Could you check a few things on this model? Use its own coordinates, in mm. A direction names the side the tool comes from. Round coordinates to 2 decimals unless told otherwise and drop trailing zeros. Write each loop counter-clockwise with the first axis right and the second up, starting at its lowest first coordinate (ties: lowest second). Pieces come first, ordered by that corner, then holes.
```python
from build123d import *

# Parameters (mm, degrees)
EXTRUDE_1_DEPTH        = 65
EXTRUDE_2_DEPTH        = 5
EXTRUDE_3_DEPTH        = 8
SKETCH_8_R             = 2.3
CUT_EXTRUDE_4_DEPTH    = 3.5
CUT_EXTRUDE_6_DEPTH    = 14
EXTRUDE_4_DEPTH        = 40
HOLE_WIZARD_M4_1_D     = 4.5
HOLE_WIZARD_M4_1_DEPTH = 10
HOLE_WIZARD_M4_1_TIP   = 1.351936393
CUT_EXTRUDE_START      = -2
SKETCH_16_R            = 3.75
CUT_EXTRUDE_7_DEPTH    = 33.495632075
F_4_0MM_1_D            = 4.55
F_4_0MM_1_DEPTH        = 3.5
CUT_EXTRUDE_8_DEPTH    = 5


with BuildPart() as part:
    # ｽｹｯﾁ1 → ﾎﾞｽ - 押し出し1 (new body)
    with BuildSketch(Plane.XY):
        Polygon((0, 0), (5.13030215, 14.095389312), (-8.965087162, 19.225691462), (-7.254986445, 23.924154566), (53.707680142, 23.924154566), (53.707680142, 18.924154566), (4.698463104, -1.710100717), align=None)
    extrude(amount=EXTRUDE_1_DEPTH)

    # ｽｹｯﾁ6 → ﾎﾞｽ - 押し出し2 (add)
    with BuildSketch(Plane(origin=(0, 0, 0), x_dir=(-1, 0, 0), z_dir=(0, 0, -1))):
        Polygon((-53.707680142, 33.124154566), (-53.707680142, 18.924154566), (-4.698463104, -1.710100717), (0, 0), (-5.13030215, 14.095389312), (8.965087162, 19.225691462), (3.90646029, 33.124154566), align=None)
    extrude(amount=EXTRUDE_2_DEPTH)

    # ｽｹｯﾁ7 → ﾎﾞｽ - 押し出し3 (add)
    with BuildSketch(Plane.XY):
        Polygon((-3.90646029, 33.124154566), (-5.726311461, 28.124154566), (53.707680142, 28.124154566), (53.707680142, 33.124154566), align=None)
    extrude(amount=EXTRUDE_3_DEPTH)

    # ｽｹｯﾁ8 → ｶｯﾄ - 押し出し4 (cut)
    with BuildSketch(Plane(origin=(0, 23.924154566, 0), x_dir=(1, 0, 0), z_dir=(0, 1, 0))):
        with Locations((7.695013555, -35)):
            Circle(SKETCH_8_R)
    extrude(amount=-CUT_EXTRUDE_4_DEPTH, mode=Mode.SUBTRACT)

    # ｽｹｯﾁ12 → ｶｯﾄ - 押し出し6 (cut, through all)
    with BuildSketch(Plane.XY.offset(8)):
        Polygon((-3.90646029, 33.124154566), (-7.254986445, 23.924154566), (11.09353971, 23.924154566), (11.09353971, 33.124154566), align=None)
    extrude(amount=-CUT_EXTRUDE_6_DEPTH, mode=Mode.SUBTRACT)

    # ｽｹｯﾁ13 → ﾎﾞｽ - 押し出し4 (add)
    with BuildSketch(Plane(origin=(0, 0, -5), x_dir=(-1, 0, 0), z_dir=(0, 0, -1))):
        Polygon((-4.698463104, -1.710100717), (0, 0), (-5.13030215, 14.095389312), (8.965087162, 19.225691462), (7.254986445, 23.924154566), (-53.707680142, 23.924154566), (-53.707680142, 18.924154566), align=None)
    extrude(amount=EXTRUDE_4_DEPTH)

    # M4 すきま穴1
    with Locations(Plane(origin=(5.13030215, 14.095389312, 0), x_dir=(-0.939692621, 0.342020143, 0), z_dir=(-0.342020143, -0.939692621, 0))):
        with Locations((7.5, -57.5), (7.5, 37.5)):
            Hole(HOLE_WIZARD_M4_1_D / 2, depth=HOLE_WIZARD_M4_1_DEPTH)
            with Locations((0, 0, -(HOLE_WIZARD_M4_1_DEPTH + HOLE_WIZARD_M4_1_TIP / 2))):  # 118° drill point
                Cone(0, HOLE_WIZARD_M4_1_D / 2, HOLE_WIZARD_M4_1_TIP, mode=Mode.SUBTRACT)

    # ｽｹｯﾁ16 → ｶｯﾄ - 押し出し7 (cut, through all)
    with BuildSketch(Plane(origin=(5.13030215, 14.095389312, 0), x_dir=(0.939692621, -0.342020143, 0), z_dir=(-0.342020143, -0.939692621, 0)).offset(CUT_EXTRUDE_START)):
        with Locations((-7.5, 57.5)):
            Circle(SKETCH_16_R)
        with Locations((-7.5, -37.5)):
            Circle(SKETCH_16_R)
    extrude(amount=-CUT_EXTRUDE_7_DEPTH, mode=Mode.SUBTRACT)

    # Ø4.0mm ﾀﾞｳｴﾙ穴1
    with Locations(Plane(origin=(0, 23.924154566, 0), x_dir=(1, 0, 0), z_dir=(0, 1, 0))):
        with Locations((28.707680142, 37.5), (28.707680142, 12.5)):
            Hole(F_4_0MM_1_D / 2, depth=F_4_0MM_1_DEPTH)

    # ｽｹｯﾁ19 → ｶｯﾄ - 押し出し8 (cut)
    with BuildSketch(Plane(origin=(53.707680142, 0, 0), x_dir=(0, 0, -1), z_dir=(1, 0, 0))):
        Polygon((0, 23.924154566), (5, 23.924154566), (5, 33.124154566), (-8, 33.124154566), (-8, 28.124154566), (0, 28.124154566), align=None)
    extrude(amount=-CUT_EXTRUDE_8_DEPTH, mode=Mode.SUBTRACT)


solid = part.part
```
Q1. We'd pull the mould along Z, two halves only. Please class faces 4 (the cylindrical face through (-1.85, 17.71, -39.73)), 5 (the flat face through (2.382, -0.867, 10.77)), 6 (the flat face through (30, 31, 8)): pulls with the +Z half, pulls with the -Z half, needs draft (parallel to the pull), parting line crosses it, or undercut.
Q2. Imagine slicing it at C-C, the plane x = 34. Write out the boundary of the cut face in (y, z), then the cut area to 3 significant figures.
Q3. Imagine slicing it at B-B, the plane z = -28.5. Write out the boundary of the cut face in (x, y), then the cut area to 3 significant figures.
Q4. Imagine slicing it at A-A, the plane z = 4. Write out the boundary of the cut face in (x, y).
Q5. If I drill on L1, parallel to Z at x = -3, y = 19.5; L2, parallel to X at y = 22.5, z = -37.5; L3, parallel to Z at x = 28, y = 23, over which ranges is the centre line in solid material (lowest first)?
Q6. Imagine slicing it at D-D, the plane z = 35. Write out the boundary of the cut face in (x, y).
Q7. I'm going to push flat-ended pins straight in: pin 1 Ø5.5 at (x, y) = (21.5, 31.5) entering from +Z; pin 2 Ø4 at (x, z) = (35, 42) entering from +Y; pin 3 Ø10 at (y, z) = (30, 3) entering from +X; pin 4 Ø8 at (y, z) = (23, 1) entering from -X. Where does each tip first touch, or does it pass through?
Q8. On a 3-axis mill with a long thin cutter (end or side, diameter ignored), from which of +Z, -Z, +X, -X, +Y, -Y can I reach the whole of each face in a straight line? I mean faces 1 (the flat face through (2.53, 6.95, 10.77)), 2 (the flat face through (30, 29, -5)), 3 (the flat face through (8, 20.424, 35)). Say none if no direction works.
Results found:
1. face 4: undercut
1. face 5: needs draft
1. face 6: pulls with the +Z half
2. outline: (10.63, -45) - (23.92, -45) - (23.92, -5) - (33.12, -5) - (33.12, 8) - (28.12, 8) - (28.12, 0) - (23.92, 0) - (23.92, 65) - (10.63, 65) - close
2. area: 1,550 mm2
3. outline: (-8.97, 19.23) - (5.13, 14.1) - (0, 0) - (4.7, -1.71) - (53.71, 18.92) - (53.71, 23.92) - (-7.25, 23.92) - close
3. area: 879 mm2
4. outline: (-8.97, 19.23) - (5.13, 14.1) - (0, 0) - (4.7, -1.71) - (53.71, 18.92) - (53.71, 23.92) - (-7.25, 23.92) - close; (11.09, 28.12) - (48.71, 28.12) - (48.71, 33.12) - (11.09, 33.12) - close
5. L1: z = -45 to -40.68, -34.32 to 54.32, 60.68 to 65
5. L2: x = -7.77 to -3.78, 4.2 to 26.43, 30.98 to 53.71
5. L3: z = -45 to -39.66, -35.34 to -14.66, -10.34 to 65
6. outline: (-8.97, 19.23) - (5.13, 14.1) - (0, 0) - (4.7, -1.71) - (53.71, 18.92) - (53.71, 23.92) - (10, 23.92) - (10, 20.42) - (5.4, 20.42) - (5.4, 23.92) - (-7.25, 23.92) - close
7. pin 1: stops at z = 8
7. pin 2: stops at y = 23.92
7. pin 3: stops at x = 48.71
7. pin 4: stops at x = -8.97
8. face 1: +Z, -Z, -X
8. face 2: -Z, +X, -X, +Y
8. face 3: +Y
